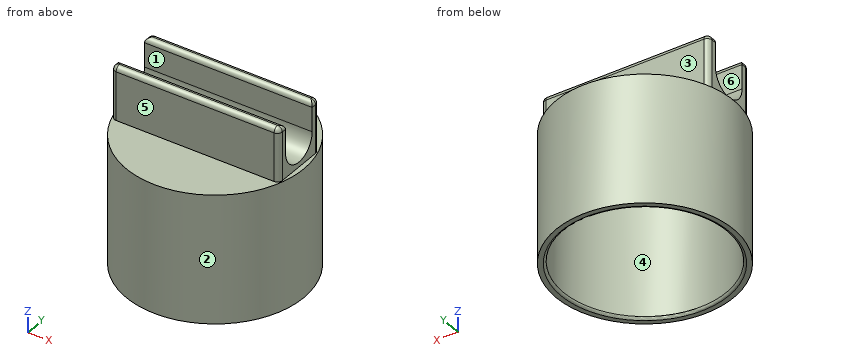
```python
from build123d import *

# Parameters (mm, degrees)
F0_R         = 18.3
F0_R_2       = 16.8
F1_DEPTH     = 25
F2_R         = 18.3
F2_R_2       = 16.8
F3_DEPTH     = 1.5
F4_W         = 34.5768708821
F4_H         = 12
F5_DEPTH     = 5
F7_DEPTH     = 36
F8_W         = 34.5768708821
F8_H         = 2
F7_FACE_W    = 34.5768708821
F7_FACE_H    = 2
F9_DEPTH     = 6
F10_R        = 0.99999
F11_T1_DEPTH = 11
F11_T4_ANGLE = 90
F12_R        = 0.5


# Not quite as in the source:
# - a fillet or chamfer that OpenCascade refuses, or shapes differently, is made with other operations: its cross-section is extruded or revolved along the edge and cut away or added
# - a fillet or chamfer is up to 0.001 mm smaller than in the source, because OpenCascade refuses the exact size


with BuildPart() as f1:
    # F0 (on Top) → F1 (new body)
    with BuildSketch(Plane.XY):
        Circle(F0_R)
        Circle(F0_R_2, mode=Mode.SUBTRACT)
    extrude(amount=F1_DEPTH)

    # F2 (on face) → F3 (join)
    with BuildSketch(Plane.XY.offset(25)):
        Circle(F2_R)
        Circle(F2_R_2, mode=Mode.SUBTRACT)
        Circle(F2_R_2)
    extrude(amount=F3_DEPTH)

    # F4 (on face) → F5 (join)
    with BuildSketch(Plane.XY.offset(26.5)):
        Rectangle(F4_W, F4_H)
    extrude(amount=F5_DEPTH)

    # F6 (on face) → F7 (cut)
    with BuildSketch(Plane.YZ.offset(17.2884354411)):
        with BuildLine():
            ThreePointArc((-4, 31.5), (0, 27.5), (4, 31.5))
            Line((4, 31.5), (-4, 31.5))
        make_face()
    extrude(amount=-F7_DEPTH, mode=Mode.SUBTRACT)

    # F8 (on face) + F7_face (on face) → F9 (join)
    with BuildSketch(Plane.XY.offset(31.5)):
        with Locations((0, -5)):
            Rectangle(F8_W, F8_H)
    with BuildSketch(Plane(origin=(0, -5, 31.5), x_dir=(1, 0, 0), z_dir=(0, 0, 1))):
        with Locations((0, 10)):
            Rectangle(F7_FACE_W, F7_FACE_H)
    extrude(amount=F9_DEPTH)

    # F10 (radius 1 in the source; OpenCascade refuses exactly that, so slightly less here)
    f10_edges = [f1.edges().sort_by_distance(p)[0] for p in [
        (17.288435, -5, 37.5),
        (0, -4, 37.5),
        (-17.288435, -5, 37.5),
        (0, -6, 37.5),
        (-17.288435, 5, 37.5),
        (0, 4, 37.5),
        (17.288435, 5, 37.5),
        (0, 6, 37.5),
        (17.288435, -6, 32),
        (-17.288435, -6, 32),
        (-17.288435, 6, 32),
    ]]
    fillet(f10_edges, radius=F10_R)

    # F11: fillet of radius 1 on 1 edges, made by hand

    # F11_s2 → F11_t1 (cut)
    with BuildSketch(Plane.XY.offset(26.5)):
        with BuildLine():
            ThreePointArc((17.2884354411, 5), (16.9955422223, 5.7071067812), (16.2884354411, 6))
            Line((16.2884354411, 6), (17.2884354411, 6))
            Line((17.2884354411, 6), (17.2884354411, 5))
        make_face()
    extrude(amount=F11_T1_DEPTH, mode=Mode.SUBTRACT)

    # F11_s3 → F11_t4 (revolve, cut)
    with BuildSketch(Plane.XZ.offset(-5)):
        with BuildLine():
            ThreePointArc((16.2884454411, 37.5), (16.9955451512, 37.2071097101), (17.2884354411, 36.50001))
            Line((17.2884354411, 36.50001), (17.2884354411, 37.5))
            Line((17.2884354411, 37.5), (16.2884454411, 37.5))
        make_face()
    revolve(axis=Axis((16.2884354411, 5, 37.5), (0, 0, 1)), revolution_arc=F11_T4_ANGLE, mode=Mode.SUBTRACT)

    # F12
    f12_edges = [f1.edges().sort_by_distance(p)[0] for p in [
        (-16.8, 0, 0),
    ]]
    fillet(f12_edges, radius=F12_R)


solid = f1.part
```
Could you check a few things on this model? Use its own coordinates, in mm. Face numbers are marked on the shaded views. A direction names the side the tool comes from. Round coordinates to 2 decimals unless told otherwise and drop trailing zeros. Write each loop counter-clockwise with the first axis right and the second up, starting at its lowest first coordinate (ties: lowest second). Pieces come first, ordered by that corner, then holes. Notation, with made-up numbers: M -10.5,52.25 L 41.5,52.25 A27 cw 41.5,89.25 Z; hole C 57.25,43.5 d6. An arc over 180 degrees is marked long. Write each question's results on one line, items separated by ' | '. Start each with the question number.
1. Imagine slicing it at C-C on y = 0. List the corners of the cut face in (x, z) for me, and give its area (3 significant figures).
2. Imagine slicing it at D-D on z = 15.5. List the corners of the cut face in (x, y) for me.
3. On a 3-axis mill with a long thin cutter (end or side, diameter ignored), from which of +Z, -Z, +X, -X, +Y, -Y can I reach the whole of each face in a straight line? I mean the marked faces 4, 5 and 6. Say none if no direction works.
4. I'm going to push flat-ended pins straight in: pin 1 Ø12 at (y, z) = (-8, 29) entering from -X; pin 2 Ø4 at (x, y) = (1.5, -9) entering from -Z; pin 3 Ø1 at (y, z) = (2.5, 26) entering from -X; pin 4 Ø4 at (x, y) = (11, 3) entering from +Z. Where does each tip first touch, or does it pass through?
5. Imagine slicing it at A-A on z = 35.5. List the corners of the cut face in (x, y) for me, and give its area (3 significant figures).
6. Thinking about a two-plate mould opening in Y: for the marked faces 1, 2 and 3, which applies, +Y half, -Y half, draft (parallel to the pull), parting line (faces both ways), or undercut?
7. I need wall thicknesses on L1, parallel to Y at x = 0.5, z = 14.5; L2, parallel to Y at x = -10, z = 35; L3, parallel to Z at x = -1, y = 5. Which ranges of each line are inside material? Lowest first, please. Write a range as from..to.
Result sheet:
1) outline: M -18.3,0 L -17.3,0 A0.5 ccw -16.8,0.5 L -16.8,25 L 16.8,25 L 16.8,0.5 A0.5 ccw 17.3,0 L 18.3,0 L 18.3,26.5 L 17.29,26.5 L 17.29,27.5 L -17.29,27.5 L -17.29,26.5 L -18.3,26.5 Z | area: 164 mm^2
2) outline: C 0,0 d36.6; hole C 0,0 d33.6
3) face 4: -Z | face 5: +Z, +X, -X, -Y | face 6: +Z, +X, -X
4) pin 1: stops at x = -18.12 | pin 2: stops at z = 25 | pin 3: stops at x = -18.19 | pin 4: stops at z = 37.5
5) outline: M -17.29,-5 A1 ccw -16.29,-6 L 16.29,-6 A1 ccw 17.29,-5 L 17.29,-4 L -17.29,-4 Z; M -17.29,4 L 17.29,4 L 17.29,5 A1 ccw 16.29,6 L -16.29,6 A1 ccw -17.29,5 Z | area: 137 mm^2
6) face 1: undercut | face 2: parting line | face 3: +Y half
7) L1: y = -18.29..-16.79, 16.79..18.29 | L2: y = -6..-4, 4..6 | L3: z = 25..37.5
